Here's how the part is built. I have some questions about the finished solid (model axes, mm). Face numbers are marked on the shaded views. A direction names the side the tool comes from. Coordinates: 2 decimals unless noted, no trailing zeros. Write each loop counter-clockwise with the first axis right and the second up, starting at its lowest first coordinate (ties: lowest second). Pieces come first, ordered by that corner, then holes.
Item 1: If we section it at A-A (y = -77): Please give me the cut outline in (x, z), then the cut area to 3 significant figures.
Item 2: If we section it at B-B (z = 29): Please give me the cut outline in (x, y), then the cut area to 3 significant figures.
Item 3: If we section it at C-C (x = 37.5): Please give me the cut outline in (y, z), then the cut area to 3 significant figures.
Item 4: For the marked faces 1 and 2, which set-ups out of +Z, -Z, +X, -X, +Y, -Y let a thin tool reach every point of the face, with its end or its side?
Item 5: If I drill on line 1 (Z direction, x = 32, y = -45); line 2 (Z direction, x = 20, y = -83), over which ranges is the centre line in solid material (lowest first)?
Item 6: I'm going to push flat-ended pins straight in: pin 1 Ø21 at (y, z) = (-69.5, 28) entering from +X; pin 2 Ø6 at (x, y) = (35, -64) entering from +Z. Where does each tip first touch, or does it pass through?
from build123d import *

# Parameters (mm, degrees)
PAD_DEPTH = 100


with BuildPart() as part:
    # Sketch → Pad (new body)
    with BuildSketch(Plane.XZ):
        with BuildLine():
            Line((0, 0), (0, 40))
            Line((0, 40), (15, 40))
            Line((15, 40), (15, 21))
            ThreePointArc((15, 21), (16.757359, 16.757359), (21, 15))
            Line((21, 15), (40, 15))
            Line((40, 15), (40, 0))
            Line((40, 0), (0, 0))
        make_face()
    extrude(amount=PAD_DEPTH)


solid = part.part
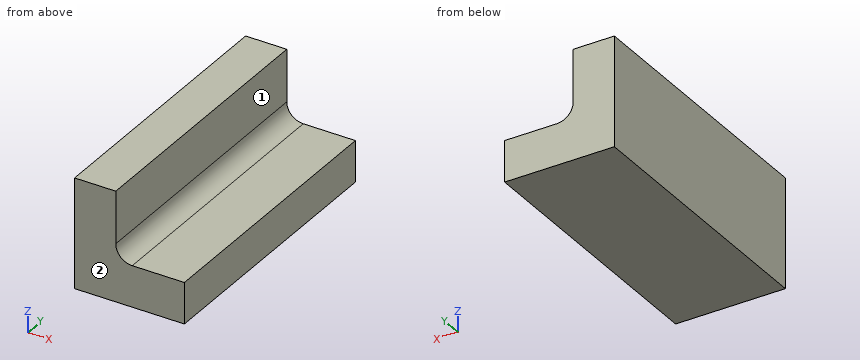
Answer list:
1. outline: (0, 0) - (40, 0) - (40, 15) - (21, 15) arc R6 cw to (15, 21) - (15, 40) - (0, 40) - close
1. area: 983 mm2
2. outline: (0, -100) - (15, -100) - (15, 0) - (0, 0) - close
2. area: 1,500 mm2
3. outline: (-100, 0) - (0, 0) - (0, 15) - (-100, 15) - close
3. area: 1,500 mm2
4. face 1: +Z, +X, +Y, -Y
4. face 2: +Z, -Z, +X, -X, -Y
5. line 1: z = 0 to 15
5. line 2: z = 0 to 15.08
6. pin 1: stops at x = 16.13
6. pin 2: stops at z = 15
